For this review, use the dimensioned drawing (mm, ordinates from the lowest corner) and the shaded views. A direction names the side the tool comes from. Coordinates: 2 decimals unless noted, no trailing zeros. Loops run counter-clockwise (first coordinate to the right, second up) from the corner with the lowest first, then second, coordinate; pieces in that order, holes last. Notation, with made-up numbers: (48.25, 23) - (105.25, 23) arc R6 cw to (105.25, 34) - close; hole circle Ø1 at (-35, -6.5). An arc over 180 degrees is marked (long way). Answer in a Markdown table with one row per item. Add a question column.
(1) We need section B-B on y = 39. Write out the cut boundary in (x, z) (1 decimal).
(2) We need section D-D on z = 17.75. Write out the cut boundary in (x, y).
(3) Mouldability with a two-part tool opening along X and no side actions: class the marked faces 3, 4 and 5 as +X half, -X half, draft (parallel to the pull), parting line (faces both ways), or undercut.
(4) For line 1 along Y through (x, z) = (22, 18); line 2 along Y through (x, z) = (19.5, 18.25) (1 decimal); line 3 along Z through (x, y) = (33, 4.5), list the stretches that pass through material, from the lowest coordinate up.
(5) For P1, Ø2, axis at y = 27.5, z = 21.5, coming from the -X side; P2, Ø4, axis at y = 37, z = 18.5, coming from the +X side; P3, Ø3, axis at y = 32.5, z = 12.5, coming from the +X side (1 decimal); P4, Ø1, axis at x = 17.5, y = 36.5, coming from the -Z side, all flat-tipped, find the tip position at first contact; note any pin that passes through.
(6) We need section C-C on y = 22. Write out the cut boundary in (x, z).
(7) Machinability: for the marked faces 1 and 2, which of the approach directions +Z, -Z, +X, -X, +Y, -Y give a long, thin tool a straight path to every point of the face, cutting with its end or side? Answer none if there is none.
(8) We need section A-A on x = 22. Write out the cut boundary in (y, z), plus the area to 3 significant figures.
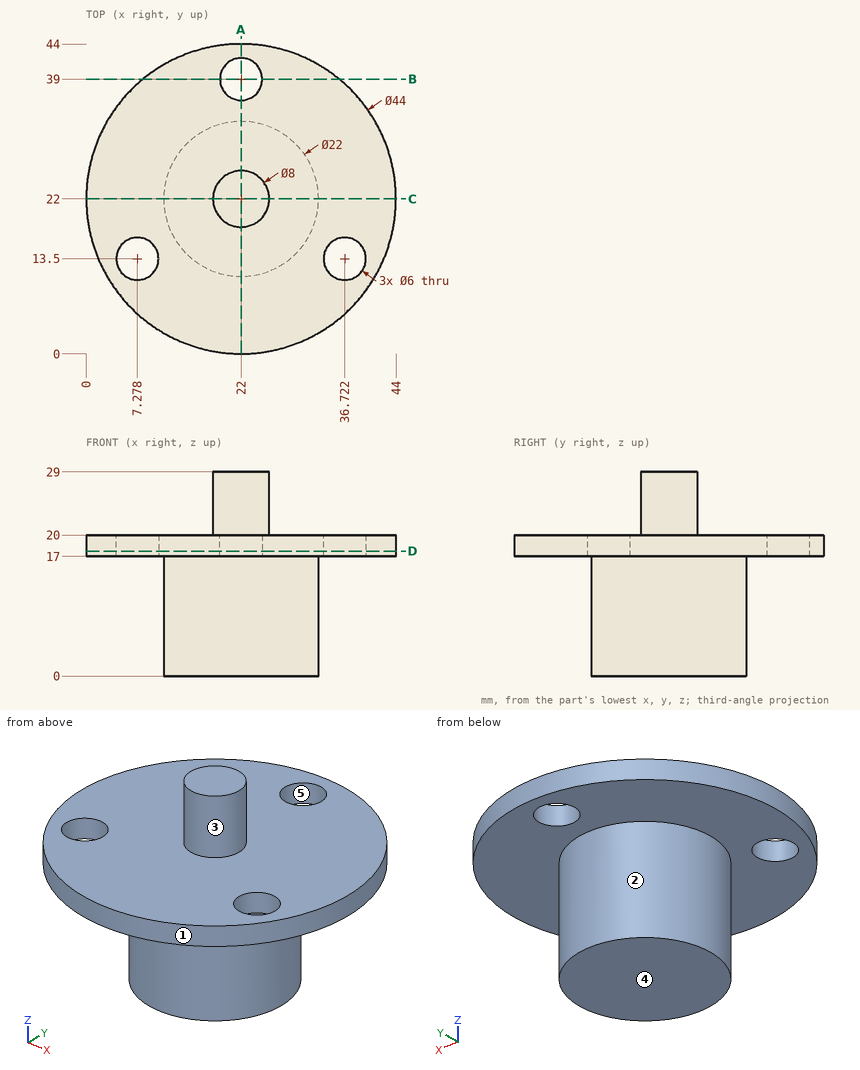
Outcome:
| question | item | result |
|---|---|---|
| 1 | outline | (8, 17) - (19, 17) - (19, 20) - (8, 20) - close; (25, 17) - (36, 17) - (36, 20) - (25, 20) - close |
| 2 | outline | circle Ø44 at (22, 22); hole circle Ø6 at (7.28, 13.5); hole circle Ø6 at (22, 39); hole circle Ø6 at (36.72, 13.5) |
| 3 | face 3 | parting line |
| 3 | face 4 | draft |
| 3 | face 5 | undercut |
| 4 | line 1 | 0 to 36, 42 to 44 |
| 4 | line 2 | 0.1 to 37.3, 40.7 to 43.9 |
| 4 | line 3 | 17 to 20 |
| 5 | P1 | through |
| 5 | P2 | x = 39.75 |
| 5 | P3 | x = 28.3 |
| 5 | P4 | z = 17 |
| 6 | outline | (0, 17) - (11, 17) - (11, 0) - (33, 0) - (33, 17) - (44, 17) - (44, 20) - (26, 20) - (26, 29) - (18, 29) - (18, 20) - (0, 20) - close |
| 7 | face 1 | +Z, -Z |
| 7 | face 2 | -Z |
| 8 | outline | (0, 17) - (11, 17) - (11, 0) - (33, 0) - (33, 17) - (36, 17) - (36, 20) - (26, 20) - (26, 29) - (18, 29) - (18, 20) - (0, 20) - close; (42, 17) - (44, 17) - (44, 20) - (42, 20) - close |
| 8 | area | 560 mm² |
